Autodesk Inventor part; units mm, degrees
ref_plane "YZ Plane" through (0, 0, 0) normal (1, 0, 0) x (0, 1, 0)
ref_plane "XZ Plane" through (0, 0, 0) normal (0, 1, 0) x (-1, 0, 0)
ref_plane "XY Plane" through (0, 0, 0) normal (0, 0, 1) x (1, 0, 0)
sketch "Skizze1" plane through (0, 0, 0) normal (0, 0, 1) x (1, 0, 0)
  circle A0 centre (0, 0) radius 6
  circle A1 centre (0, 0) radius 3.05
  dimension "d0" = 6.1
  dimension "d1" = 12
extrude "Extrusion1" add sketch "Skizze1" along normal blind 2
sketch "Skizze2" plane through (0, 0, 2) normal (0, 0, 1) x (1, 0, 0)
  circle A0 centre (0, 0) radius 6
extrude "Extrusion2" add sketch "Skizze2" along normal blind 0.2
sketch "Skizze3" plane through (0, 0, 2.2) normal (0, 0, 1) x (1, 0, 0)
  circle A0 centre (0, 0) radius 6
  line L0 (0, 4.6188) -> (4, 2.3094)
  line L1 (4, 2.3094) -> (4, -2.3094)
  line L2 (4, -2.3094) -> (0, -4.6188)
  line L3 (0, -4.6188) -> (-4, -2.3094)
  line L4 (-4, -2.3094) -> (-4, 2.3094)
  line L5 (-4, 2.3094) -> (0, 4.6188)
  dimension "d6" = 8
extrude "Extrusion3" add sketch "Skizze3" along normal blind 3
properties part number "M5_encoderMagnet" material "ABS-Kunststoff - Schwarz"
CAD build for the part. Positions are in the model's coordinates, mm. A direction names the side the tool comes from. Round coordinates to 2 decimals unless told otherwise and drop trailing zeros. Loops run counter-clockwise (first coordinate to the right, second up) from the corner with the lowest first, then second, coordinate; pieces in that order, holes last.
(1) Cut at C-C (x = 2.25). Give the cut face in (y, z), plus the area to 3 significant figures.
(2) Two-plate mould, pull along Y, no slides. Class faces 1 (the flat face through (-1.4, 4.1, 5.2)), 2 (the cylindrical face through (-6, 0, 3)), 3 (the flat face through (4, 0, 4)), 4 (the flat face through (-4, 0, 4)): +Y half, -Y half, draft (parallel to the pull), parting line (faces both ways), or undercut.
(3) Cut at B-B (y = 0). Give the cut face in (x, z).
(4) Wall check: line 1 along Y through (x, z) = (0, 1.2); line 2 along Z through (x, y) = (1.75, 1.5); line 3 along X through (y, z) = (2.25, 4.75). Give the ranges that are in metal, low to high.
(5) Cut at A-A (z = 4.05). Give the cut face in (x, y), plus the area to 3 significant figures.
(6) Cut at D-D (z = 1.2). Give the cut face in (x, y), plus the area to 3 significant figures.
(7) Drop flat-ended pins along their axis: pin 1 (6 mm diameter, centred on x = -0.5, y = -1.5, fed in from -Z); pin 2 (0.9 mm diameter, centred on y = 1, z = 3.5, fed in from +X); pin 3 (3 mm diameter, centred on x = 5, z = 2, fed in from +Y); pin 4 (3 mm diameter, centred on x = -2.5, z = 4.5, fed in from -Y). Give the stop position or say it passes through.
(8) Which spindle directions (+Z, -Z, +X, -X, +Y, -Y) get a long thin tool onto all of the face, cutting with end or side? Do faces 5 (the flat face through (0, 0, 2)), 6 (the flat face through (-2.028, 3.448, 3.679)), 7 (the flat face through (3, -3, 0)). Say none if no direction does.
Findings below:
1. outline: (-5.56, 0) - (-2.06, 0) - (-2.06, 2) - (2.06, 2) - (2.06, 0) - (5.56, 0) - (5.56, 5.2) - (3.32, 5.2) - (3.32, 2.2) - (-3.32, 2.2) - (-3.32, 5.2) - (-5.56, 5.2) - close
1. area: 29.7 mm2
2. face 1: draft
2. face 2: parting line
2. face 3: undercut
2. face 4: undercut
3. outline: (-6, 0) - (-3.05, 0) - (-3.05, 2) - (3.05, 2) - (3.05, 0) - (6, 0) - (6, 5.2) - (4, 5.2) - (4, 2.2) - (-4, 2.2) - (-4, 5.2) - (-6, 5.2) - close
4. line 1: y = -6 to -3.05, 3.05 to 6
4. line 2: z = 2 to 2.2
4. line 3: x = -5.56 to -4, 4 to 5.56
5. outline: circle Ø12 at (0, 0); hole (-4, -2.31) - (0, -4.62) - (4, -2.31) - (4, 2.31) - (0, 4.62) - (-4, 2.31) - close
5. area: 57.7 mm2
6. outline: circle Ø12 at (0, 0); hole circle Ø6.1 at (0, 0)
6. area: 83.9 mm2
7. pin 1: stops at z = 0
7. pin 2: stops at x = 5.97
7. pin 3: stops at y = 4.87
7. pin 4: stops at y = -5.92
8. face 5: -Z
8. face 6: +Z
8. face 7: -Z, +X, -X, +Y, -Y
